from build123d import *

# Parameters (mm, degrees)
BOSS_EXTRUDE1_DEPTH     = 12.5
SKETCH2_W               = 12.5
SKETCH2_H               = 2
BOSS_EXTRUDE2_DEPTH     = 6
SKETCH3_R               = 1.25
CUT_EXTRUDE1_DEPTH      = 32.713927878
CUT_EXTRUDE1_DEPTH_BACK = 16.499999831
SKETCH5_W               = 8.5
SKETCH5_H               = 8.5
CUT_EXTRUDE2_DEPTH      = 26.999999831


with BuildPart() as part:
    # Sketch1 → Boss-Extrude1 (new body)
    with BuildSketch(Plane.XY):
        with BuildLine():
            ThreePointArc((8, 17), (7.694207367, 19.190701486), (6.80020675, 21.213927878))
            Line((6.80020675, 21.213927878), (4.814885895, 18.847914617))
            ThreePointArc((4.814885895, 18.847914617), (4.953505298, 18.180283222), (5, 17.5))
            Line((5, 17.5), (5, -17.5))
            ThreePointArc((5, -17.5), (0, -22.5), (-5, -17.5))
            Line((-5, -17.5), (-5, 17.5))
            Line((-5, 17.5), (-7.984359711, 17.5))
            ThreePointArc((-7.984359711, 17.5), (-7.996088972, 17.250122279), (-8, 17))
            Line((-8, 17), (-8, -17.999999662))
            ThreePointArc((-8, -17.999999662), (-1.69e-07, -25.999999831), (8, -18))
            Line((8, -18), (8, 17))
        make_face()
    extrude(amount=BOSS_EXTRUDE1_DEPTH)

    # Sketch2 → Boss-Extrude2 (add)
    with BuildSketch(Plane(origin=(8, 0, 0), x_dir=(0, 0, -1), z_dir=(1, 0, 0))):
        with Locations((-6.25, -11.5)):
            Rectangle(SKETCH2_W, SKETCH2_H)
        with Locations((-6.25, -6.5)):
            Rectangle(SKETCH2_W, SKETCH2_H)
    extrude(amount=BOSS_EXTRUDE2_DEPTH)

    # Sketch3 → Cut-Extrude1 (cut, two sides)
    with BuildSketch(Plane(origin=(0, -10.5, 0), x_dir=(1, 0, 0), z_dir=(0, 1, 0))) as cut_extrude1_sk:
        with Locations((11, -3)):
            Circle(SKETCH3_R)
        with Locations((11, -9.5)):
            Circle(SKETCH3_R)
    extrude(amount=CUT_EXTRUDE1_DEPTH, mode=Mode.SUBTRACT)
    extrude(cut_extrude1_sk.sketch, amount=-CUT_EXTRUDE1_DEPTH_BACK, mode=Mode.SUBTRACT)

    # Sketch5 → Cut-Extrude2 (cut, through all)
    with BuildSketch(Plane(origin=(0, 0, 0), x_dir=(1, 0, 0), z_dir=(0, 1, 0))):
        with Locations((0, -6.25)):
            Rectangle(SKETCH5_W, SKETCH5_H)
    extrude(amount=-CUT_EXTRUDE2_DEPTH, mode=Mode.SUBTRACT)


solid = part.part
Model file for the job. Use its own axes, mm. A direction names the side the tool comes from. Round coordinates to 2 decimals unless told otherwise and drop trailing zeros. Order: outer loops, then holes, each group sorted by start corner. A loop starts at its lowest first (then second) coordinate and runs counter-clockwise, first axis right, second up. Notation, with made-up numbers: M 71.5,-26 L 110.5,-26 A13 ccw 110.5,-12 Z; hole C 23,63.5 d7. An arc over 180 degrees is marked long. Write each question's results on one line, items separated by ' | '. Start each with the question number.
(1) Saw through at B-B, the plane y = -1. Give the cut face in (x, z).
(2) Drop flat-ended pins along their axis: pin 1 (1.5 mm diameter, centred on x = 11, z = 3, fed in from +Y); pin 2 (3 mm diameter, centred on x = 10, z = 8, fed in from +Y); pin 3 (1.8 mm diameter, centred on x = 9.5, z = 5, fed in from -Y); pin 4 (1 mm diameter, centred on x = -4, z = 5.5, fed in from +Y). Give the stop position or say it passes through.
(3) Which spindle directions (+Z, -Z, +X, -X, +Y, -Y) get a long thin tool onto all of the face, cutting with end or side? Do faces 5 (the face through (-5, 0, 6)), 6 (the face through (0, -24, 10.5)), 7 (the face through (11, -12.5, 6)), 8 (the face through (5, 0, 6)), 9 (the face through (14, -6, 6)). Say none if no direction does.
(4) Saw through at C-C, the plane x = 11. Give the cut face in (y, z).
(5) Probe probe 1 along Z at (x, y) = (11, -11.2); probe 2 along X at (y, z) = (-11.2, 9.5); probe 3 along X at (y, z) = (17, 1.25). List the from-to ranges inside material, lowest first. Write a range as from..to.
(6) Saw through at D-D, the plane z = 6.5. Give the cut face in (x, y), then the cut area to 3 significant figures.
(7) Saw through at A-A, the plane z = 9.5. State how many separate pieces and enclosed holes the cut face has, then the cut area to 3 significant figures.
(8) Two-plate mould, pull along Y, no slides. Class faces 1 (the face through (11, -7.5, 6)), 2 (the face through (-6, 17.5, 6)), 3 (the face through (8, -9, 6)), 4 (the face through (-4.25, -22, 6)): pulls with the +Y half, pulls with the -Y half, needs draft (parallel to the pull), parting line crosses it, or undercut.
Established:
1) outline: M -8,0 L -5,0 L -5,12.5 L -8,12.5 Z; M 5,0 L 8,0 L 8,12.5 L 5,12.5 Z
2) pin 1: passes through | pin 2: stops at y = -5.5 | pin 3: stops at y = -12.5 | pin 4: stops at y = -19.68
3) face 5: +Z, -Z, +Y | face 6: +Y, -Y | face 7: +Z, -Z, +X, -Y | face 8: +Z, -Z | face 9: +Z, -Z, +X, +Y, -Y
4) outline: M -12.5,0 L -10.5,0 L -10.5,1.75 L -12.5,1.75 Z; M -12.5,4.25 L -10.5,4.25 L -10.5,8.25 L -12.5,8.25 Z; M -12.5,10.75 L -10.5,10.75 L -10.5,12.5 L -12.5,12.5 Z; M -7.5,0 L -5.5,0 L -5.5,1.75 L -7.5,1.75 Z; M -7.5,4.25 L -5.5,4.25 L -5.5,8.25 L -7.5,8.25 Z; M -7.5,10.75 L -5.5,10.75 L -5.5,12.5 L -7.5,12.5 Z
5) probe 1: z = 0..1.75, 4.25..8.25, 10.75..12.5 | probe 2: x = -8..-5, 5..9.75, 12.25..14 | probe 3: x = -8..-5, 5..8
6) outline: M -8,-18 A8 ccw -4.25,-24.78 L -4.25,-20.13 A5 cw -5,-17.5 L -5,17.5 L -7.98,17.5 A8 ccw -8,17 Z; M 4.25,-24.78 A8 ccw 8,-18 L 8,-12.5 L 14,-12.5 L 14,-10.5 L 8,-10.5 L 8,-7.5 L 14,-7.5 L 14,-5.5 L 8,-5.5 L 8,17 A8 ccw 6.8,21.21 L 4.81,18.85 A5 cw 5,17.5 L 5,-17.5 A5 cw 4.25,-20.13 Z | area: 279 mm^2
7) separate pieces: 4 | enclosed holes: 0 | area: 269 mm^2
8) face 1: undercut | face 2: pulls with the +Y half | face 3: undercut | face 4: needs draft
